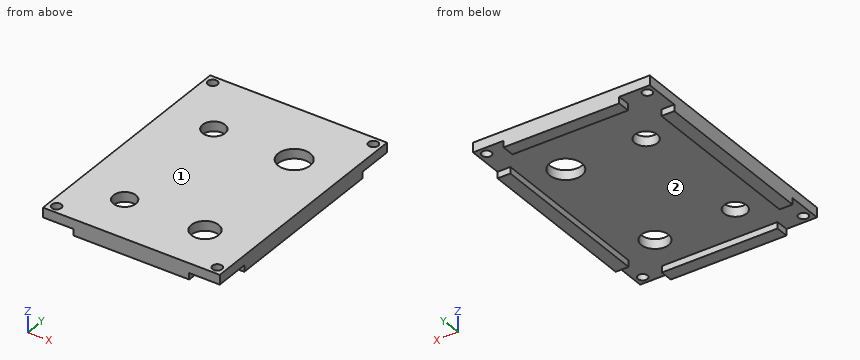
Solid Edge part; units mm, degrees
sketch "Sketch1" plane through (0, 0, 0) normal (0, 0, 1) x (1, 0, 0)
  circle A0 centre (15.8237, 56) radius 3.5
  circle A1 centre (15.8237, 16) radius 3.5
  circle A2 centre (40.8237, 16) radius 4.25
  circle A3 centre (40.8237, 56) radius 5
  line L0 (0.8237, 1) -> (0.8237, 76)
  line L1 (0.8237, 76) -> (55.8237, 76)
  line L2 (55.8237, 76) -> (55.8237, 1)
  line L3 (55.8237, 1) -> (0.8237, 1)
  circle A4 centre (3.3237, 73.5) radius 1.5
  circle A5 centre (53.3237, 73.5) radius 1.5
  circle A6 centre (3.3237, 3.5) radius 1.5
  circle A7 centre (53.3237, 3.5) radius 1.5
extrude "Protrusion1" add sketch "Sketch1" along normal blind 3
sketch "Sketch2" plane through (0, 0, 0) normal (0, 0, 1) x (1, 0, 0)
  line L0 (46.3237, 72) -> (10.3237, 72)
  line L1 (10.3237, 72) -> (10.3237, 76)
  line L2 (10.3237, 76) -> (46.3237, 76)
  line L3 (46.3237, 76) -> (46.3237, 72)
  line L4 (0.8237, 65) -> (4.8237, 65)
  line L5 (4.8237, 65) -> (4.8237, 12)
  line L6 (4.8237, 12) -> (0.8237, 12)
  line L7 (0.8237, 12) -> (0.8237, 65)
  line L8 (55.8237, 65) -> (51.8237, 65)
  line L9 (51.8237, 65) -> (51.8237, 12)
  line L10 (51.8237, 12) -> (55.8237, 12)
  line L11 (55.8237, 12) -> (55.8237, 65)
  line L12 (46.3237, 5) -> (10.3237, 5)
  line L13 (10.3237, 5) -> (10.3237, 1)
  line L14 (10.3237, 1) -> (46.3237, 1)
  line L15 (46.3237, 1) -> (46.3237, 5)
extrude "ExtrudedProtrusion_3" add sketch "Sketch2" against normal blind 2
Check sheet for the modelled part. Datum: model origin and axes. Units: mm. Face numbers are marked on the shaded views. Give positions to 0.01 mm unless a question says otherwise; leave off trailing zeros. Loops run counter-clockwise (first coordinate to the right, second up) from the corner with the lowest first, then second, coordinate; pieces in that order, holes last. Notation, with made-up numbers: M 59,59 L 66,59 A18 ccw 66,64 Z; hole C 53,-32 d8. An arc over 180 degrees is marked long. Answer in a Markdown table with one row per item.
1) Cross-section at B-B (z = 1.25). Count the separate pieces of the cut face and the enclosed holes in it, plus the area to 3 significant figures.
Solutions:
| item | result |
|---|---|
| separate pieces | 1 |
| enclosed holes | 8 |
| area | 3,880 mm^2 |
2) Cross-section at A-A (y = 56). Enter the section's corners in (x, z).
Solutions:
| item | result |
|---|---|
| outline | M 0.82,-2 L 4.82,-2 L 4.82,0 L 12.32,0 L 12.32,3 L 0.82,3 Z; M 19.32,0 L 35.82,0 L 35.82,3 L 19.32,3 Z; M 45.82,0 L 51.82,0 L 51.82,-2 L 55.82,-2 L 55.82,3 L 45.82,3 Z |
3) Thickness scan on line 1 (Y direction, x = 45.5, z = -0.95); line 2 (X direction, y = 73.5, z = 1.35); line 3 (X direction, y = 40.5, z = -1.25). Record the ranges inside material, lowest first.
Solutions:
| item | result |
|---|---|
| line 1 | y = 1 to 5, 72 to 76 |
| line 2 | x = 0.82 to 1.82, 4.82 to 51.82, 54.82 to 55.82 |
| line 3 | x = 0.82 to 4.82, 51.82 to 55.82 |
4) Depth check by flat-ended pin: pin 1 (2.5 mm diameter, centred on x = 3.32, y = 3.5, fed in from -Z); pin 2 (1.6 mm diameter, centred on x = 2.5, z = -1, fed in from +Y); pin 3 (1 mm diameter, centred on y = 3.5, z = -1.5, fed in from -X); pin 4 (8 mm diameter, centred on x = 15.82, y = 56, fed in from -Z). Enter the tip coordinate at first touch or a pass-through.
Solutions:
| item | result |
|---|---|
| pin 1 | passes through |
| pin 2 | stops at y = 65 |
| pin 3 | stops at x = 10.32 |
| pin 4 | stops at z = 0 |
5) Cross-section at C-C (x = 34). Enter the section's corners in (y, z), plus the area to 3 significant figures.
Solutions:
| item | result |
|---|---|
| outline | M 1,-2 L 5,-2 L 5,0 L 72,0 L 72,-2 L 76,-2 L 76,3 L 1,3 Z |
| area | 241 mm^2 |
6) Mould release check, pull along Y, two halves, no side actions. Record for the marked faces 1 and 2: released by +Y, released by -Y, zero draft, split by the parting line, or undercut.
Solutions:
| item | result |
|---|---|
| face 1 | zero draft |
| face 2 | undercut |
7) Cross-section at D-D (x = 14.5). Enter the section's corners in (y, z).
Solutions:
| item | result |
|---|---|
| outline | M 1,-2 L 5,-2 L 5,0 L 12.76,0 L 12.76,3 L 1,3 Z; M 19.24,0 L 52.76,0 L 52.76,3 L 19.24,3 Z; M 59.24,0 L 72,0 L 72,-2 L 76,-2 L 76,3 L 59.24,3 Z |
